from build123d import *

# Parameters (mm, degrees)
BOSS_EXTRUDE1_DEPTH        = 6
DOVE_BOSS_DEPTH            = 30
BOSS_EXTRUDE7_DEPTH        = 30
PIN_SLOT_REACH             = 39.724
PIN_SLOT_DIRECTION_2_DEPTH = 38.723710458
BOSS_EXTRUDE8_DEPTH        = 6


with BuildPart() as part:
    # Sketch1 → Boss-Extrude1 (new body)
    with BuildSketch(Plane(origin=(0, 0, 0), x_dir=(1, 0, 0), z_dir=(0, 1, 0))):
        Polygon((-30, 20), (-30, -20), (0, -20), (0, -8.167550091), (-6.853388269, 0), (0, 8.167550091), (0, 20), align=None)
        Polygon((-6.853388269, 0), (0, -8.167550091), (0, 8.167550091), align=None)
    extrude(amount=BOSS_EXTRUDE1_DEPTH)

    # Sketch7 → Dove Boss (add)
    with BuildSketch(Plane(origin=(-30, 0, 0), x_dir=(0, 0, -1), z_dir=(1, 0, 0))):
        Polygon((-12.5, 0), (-20, 0), (-22.069851171, -5), (-12.5, -5), align=None)
    extrude(amount=DOVE_BOSS_DEPTH)

    # Sketch7<3> → Boss-Extrude7 (add)
    with BuildSketch(Plane(origin=(-30, 0, 0), x_dir=(0, 0, -1), z_dir=(1, 0, 0))):
        Polygon((20, 0), (12.5, 0), (12.5, -5), (22.069851171, -5), align=None)
    extrude(amount=BOSS_EXTRUDE7_DEPTH)

    # Sketch4 → Pin Slot (cut, up to next)
    with BuildSketch(Plane(origin=(0, 0, 0), x_dir=(1, 0, 0), z_dir=(0, 1, 0)), mode=Mode.PRIVATE) as pin_slot_sk1:
        with BuildLine():
            Line((-1.5, 10), (-1.5, -10))
            ThreePointArc((-1.5, -10), (-3, -11.5), (-4.5, -10))
            Line((-4.5, -10), (-4.5, 10))
            ThreePointArc((-4.5, 10), (-3, 11.5), (-1.5, 10))
        make_face()
    pin_slot_tool1 = extrude(pin_slot_sk1.sketch, amount=PIN_SLOT_REACH, mode=Mode.PRIVATE) & part.part
    add(pin_slot_tool1.solids().sort_by_distance((-3, 0, 0))[0], mode=Mode.SUBTRACT)

    # Sketch4 → Pin Slot direction 2 (cut)
    with BuildSketch(Plane(origin=(0, 0, 0), x_dir=(1, 0, 0), z_dir=(0, 1, 0))):
        with BuildLine():
            Line((-1.5, 10), (-1.5, -10))
            ThreePointArc((-1.5, -10), (-3, -11.5), (-4.5, -10))
            Line((-4.5, -10), (-4.5, 10))
            ThreePointArc((-4.5, 10), (-3, 11.5), (-1.5, 10))
        make_face()
    extrude(amount=-PIN_SLOT_DIRECTION_2_DEPTH, mode=Mode.SUBTRACT)

    # Sketch8 → Boss-Extrude8 (add)
    with BuildSketch(Plane(origin=(0, 6, 0), x_dir=(1, 0, 0), z_dir=(0, 1, 0))):
        Polygon((0, -103.563417049), (0, -98.563417049), (-14.801872329, -85), (0, -71.436582951), (0, -20), (-19.801872329, -20), (-19.801872329, -103.563417049), align=None)
    extrude(amount=-BOSS_EXTRUDE8_DEPTH)


solid = part.part
Could you check a few things on this model? Use its own coordinates, in mm. A direction names the side the tool comes from. Round coordinates to 2 decimals unless told otherwise and drop trailing zeros. Order: outer loops, then holes, each group sorted by start corner. A loop starts at its lowest first (then second) coordinate and runs counter-clockwise, first axis right, second up.
(1) Imagine slicing it at B-B (x = -8.75). Write out the boundary of the cut face in (y, z), plus the area to 3 significant figures.
Response values:
outline: (-5, -22.07) - (0, -20) - (6, -20) - (6, 79.45) - (0, 79.45) - (0, 20) - (-5, 22.07) - (-5, 12.5) - (0, 12.5) - (0, -12.5) - (-5, -12.5) - close; (0, 90.55) - (6, 90.55) - (6, 103.56) - (0, 103.56) - close
area: 760 mm2
(2) If we mould it in two halves opening along X, with no side actions, what happens to faces 1 (the flat face through (-7.5, 3.04, 78.31)), 2 (the flat face through (-15.21, -2.535, -21.049)), 3 (the cylindrical face through (-3, 3, 11.5))? For each: released by +X, released by -X, zero draft, split by the parting line, or undercut.
Response values:
face 1: released by +X
face 2: zero draft
face 3: undercut
(3) Which directions (+Z, -Z, +X, -X, +Y, -Y) give clear straight access to the entire face, cutting with the end or side of a thin tool? Please do faces 4 (the flat face through (-7.297, 3.042, 91.877)), 5 (the cylindrical face through (-3, 3, -11.5)), 6 (the flat face through (-25, 3, 20)), 7 (the flat face through (-15, -3, 12.5)).
Response values:
face 4: +X, +Y, -Y
face 5: +Y, -Y
face 6: +Z, -X, +Y
face 7: +X, -X, -Y
(4) Imagine slicing it at A-A (y = -3.75). Write out the boundary of the cut face in (x, z), plus the area to 3 significant figures.
Response values:
outline: (-30, -21.55) - (0, -21.55) - (0, -12.5) - (-30, -12.5) - close; (-30, 12.5) - (0, 12.5) - (0, 21.55) - (-30, 21.55) - close
area: 543 mm2
(5) Imagine slicing it at C-C (x = -2.75). Write out the boundary of the cut face in (y, z).
Response values:
outline: (-5, -22.07) - (0, -20) - (6, -20) - (6, -11.48) - (0, -11.48) - (0, -12.5) - (-5, -12.5) - close; (-5, 12.5) - (0, 12.5) - (0, 11.48) - (6, 11.48) - (6, 73.96) - (0, 73.96) - (0, 20) - (-5, 22.07) - close; (0, 96.04) - (6, 96.04) - (6, 103.56) - (0, 103.56) - close
(6) Please list where these lines run through material, in increasing order: line 1 along X through (y, z) = (3.5, 10); line 2 along Y through (x, z) = (-15.25, -6.5); line 3 along X through (y, z) = (0.75, 71).
Response values:
line 1: x = -30 to -4.5, -1.5 to 0
line 2: y = 0 to 6
line 3: x = -19.8 to 0
(7) I'm going to push flat-ended pins straight in: pin 1 (5 mm diameter, centred on y = 0, z = 51.5, fed in from -X); pin 2 (3 mm diameter, centred on x = -25.5, y = 4, fed in from +Z); pin 3 (2.5 mm diameter, centred on x = -19.5, y = -2, fed in from +Z); pin 4 (8 mm diameter, centred on x = -27, z = 67.5, fed in from -Y). Where does each tip first touch, or does it pass through?
Response values:
pin 1: stops at x = -19.8
pin 2: stops at z = 20
pin 3: stops at z = 21.35
pin 4: passes through
(8) Imagine slicing it at D-D (y = 1.5). Write out the boundary of the cut face in (x, z).
Response values:
outline: (-30, -20) - (0, -20) - (0, 71.44) - (-14.8, 85) - (0, 98.56) - (0, 103.56) - (-19.8, 103.56) - (-19.8, 20) - (-30, 20) - close; hole (-4.5, -10) arc R1.5 ccw to (-1.5, -10) - (-1.5, 10) arc R1.5 ccw to (-4.5, 10) - close
